Source: CAD feature listing. Evaluate the final solid. Frame: model axes, mm. Face numbers are marked on the shaded views. A direction names the side the tool comes from. Give positions to 0.01 mm unless a question says otherwise; leave off trailing zeros. Write each loop counter-clockwise with the first axis right and the second up, starting at its lowest first coordinate (ties: lowest second). Pieces come first, ordered by that corner, then holes. Notation, with made-up numbers: (51.25, -0.75) -> (70.25, -0.75) arc R12 cw to (70.25, 4.25) -> close; hole circle Ø9 at (-0.75, 36). An arc over 180 degrees is marked (long way). Use a Markdown table: item, result. Add a question column.
```python
from build123d import *

# Parameters (mm, degrees)
F0_W     = 273.05
F0_H     = 114.3
F1_DEPTH = 19.05
F2_R     = 25.4
F3_DEPTH = 25.4
F5_DEPTH = 25.4


with BuildPart() as f1:
    # F0 (on Front) → F1 (new body)
    with BuildSketch(Plane.XZ):
        with Locations((136.525, 57.15)):
            Rectangle(F0_W, F0_H)
    extrude(amount=F1_DEPTH)

    # F2 (on face) → F3 (cut)
    with BuildSketch(Plane.XZ.offset(19.05)):
        with Locations((225.425, 50.8)):
            Circle(F2_R)
        with Locations((47.625, 50.8)):
            Circle(F2_R)
    extrude(amount=-F3_DEPTH, mode=Mode.SUBTRACT)

    # F4 (on face) → F5 (cut)
    with BuildSketch(Plane.XZ.offset(19.05)):
        with BuildLine():
            Line((177.8, 114.3), (95.25, 114.3))
            Line((95.25, 114.3), (95.25, 74.93))
            ThreePointArc((95.25, 74.93), (98.597769, 66.847769), (106.68, 63.5))
            Line((106.68, 63.5), (166.37, 63.5))
            ThreePointArc((166.37, 63.5), (174.452231, 66.847769), (177.8, 74.93))
            Line((177.8, 74.93), (177.8, 114.3))
        make_face()
    extrude(amount=-F5_DEPTH, mode=Mode.SUBTRACT)


solid = f1.part
```
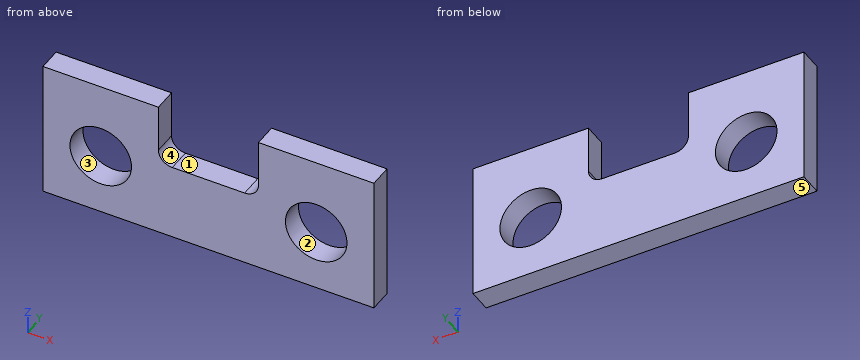
(1) Cut plane B-B on z = 84. Return the cut outline in (x, y), then the cut area to 3 significant figures.
(2) Cut plane D-D on z = 50.8. Return the cut outline in (x, y) (3 decimals), then the cut area to 3 significant figures.
(3) Material intervals for L1, parallel to X at y = -9.25, z = 57; L2, parallel to X at y = -10.5, z = 58; L3, parallel to X at y = -12.75, z = 69, sorted ascending.
(4) Access query for the marked faces 1 and 2. Directions: +Z, -Z, +X, -X, +Y, -Y. A direction counts if a zero-diameter tool reaches every point of the face in a straight line with its end or side. Return the directions, or none.
(5) First-contact query: pin 1 Ø1 at (x, y) = (104, -11.5) entering from +Z; pin 2 Ø5.5 at (x, y) = (143.5, -6) entering from +Z. Flat tips, straight axial feed; report the tip coordinate or a pass-through.
(6) Mould query, pull axis X, two halves, no side actions, for the marked faces 3, 4 and 5. Classes: +X half, -X half, draft (parallel to the pull), parting line (faces both ways), or undercut.
(7) Cut plane C-C on x = 38. Return the cut outline in (y, z).
(8) Cut plane A-A on y = -15.5. Return the cut outline in (x, z) (3 decimals).
Output:
| question | item | result |
|---|---|---|
| 1 | outline | (0, -19.05) -> (95.25, -19.05) -> (95.25, 0) -> (0, 0) -> close; (177.8, -19.05) -> (273.05, -19.05) -> (273.05, 0) -> (177.8, 0) -> close |
| 1 | area | 3,630 mm^2 |
| 2 | outline | (0, -19.05) -> (22.225, -19.05) -> (22.225, 0) -> (0, 0) -> close; (73.025, -19.05) -> (200.025, -19.05) -> (200.025, 0) -> (73.025, 0) -> close; (250.825, -19.05) -> (273.05, -19.05) -> (273.05, 0) -> (250.825, 0) -> close |
| 2 | area | 3,270 mm^2 |
| 3 | L1 | 0 to 22.99, 72.26 to 200.79, 250.06 to 273.05 |
| 3 | L2 | 0 to 23.27, 71.98 to 201.07, 249.78 to 273.05 |
| 3 | L3 | 0 to 29.91, 65.34 to 96.91, 176.14 to 207.71, 243.14 to 273.05 |
| 4 | face 1 | +Z, +Y, -Y |
| 4 | face 2 | +Y, -Y |
| 5 | pin 1 | z = 63.95 |
| 5 | pin 2 | z = 63.5 |
| 6 | face 3 | undercut |
| 6 | face 4 | undercut |
| 6 | face 5 | draft |
| 7 | outline | (-19.05, 0) -> (0, 0) -> (0, 27.29) -> (-19.05, 27.29) -> close; (-19.05, 74.31) -> (0, 74.31) -> (0, 114.3) -> (-19.05, 114.3) -> close |
| 8 | outline | (0, 0) -> (273.05, 0) -> (273.05, 114.3) -> (177.8, 114.3) -> (177.8, 74.93) arc R11.43 cw to (166.37, 63.5) -> (106.68, 63.5) arc R11.43 cw to (95.25, 74.93) -> (95.25, 114.3) -> (0, 114.3) -> close; hole circle Ø50.8 at (47.625, 50.8); hole circle Ø50.8 at (225.425, 50.8) |
